Input: part model. Units: mm. Frame: model coordinates. Give positions to 0.01 mm unless a question says otherwise; leave off trailing zeros. Loops run counter-clockwise (first coordinate to the right, second up) from the corner with the lowest first, then second, coordinate; pieces in that order, holes last. Notation, with made-up numbers: (-18.5, 51.25) -> (16.5, 51.25) arc R28 cw to (16.5, 75.25) -> close; hole circle Ø3 at (13, -36). An arc over 180 degrees is marked (long way). Answer as a JSON object with one key per item and string values. Group by question number.
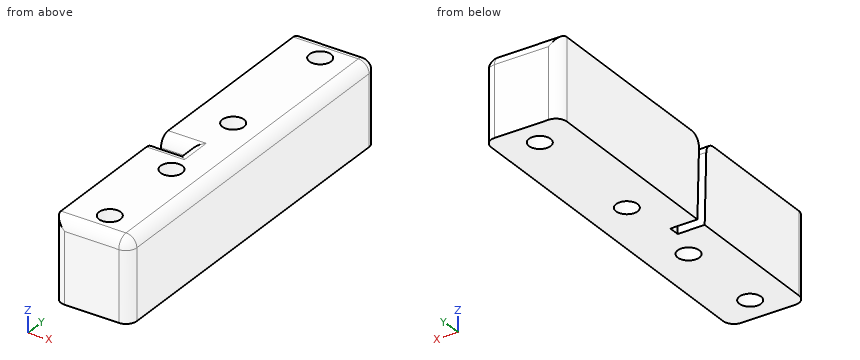
```python
from build123d import *

# Parameters (mm, degrees)
F0_W     = 14
F0_H     = 28
F0_R     = 2
F1_DEPTH = 15
F0_H_2   = 38
F2_W     = 2.6328479201
F2_H     = 15
F3_DEPTH = 9
F5_DEPTH = 5
F7_DEPTH = 5
F8_R     = 2


with BuildPart() as f1:
    # F0 (on Top) → F1 (new body)
    with BuildSketch(Plane.XY):
        with Locations((7, 14)):
            Rectangle(F0_W, F0_H)
        with Locations((7, 5)):
            Circle(F0_R, mode=Mode.SUBTRACT)
        with Locations((7, 22)):
            Circle(F0_R, mode=Mode.SUBTRACT)
    extrude(amount=F1_DEPTH)



with BuildPart() as f1b:
    # F0 (on Top) → F1, piece 2 (new body)
    with BuildSketch(Plane.XY):
        with Locations((7, 49)):
            Rectangle(F0_W, F0_H_2)
        with Locations((7, 39)):
            Circle(F0_R, mode=Mode.SUBTRACT)
        with Locations((7, 63)):
            Circle(F0_R, mode=Mode.SUBTRACT)
    extrude(amount=F1_DEPTH)


with BuildPart() as f1_1:
    add(f1.part)

    add(f1b.part)  # F3 merges F1b
    # F2 (on face) → F3 (join)
    with BuildSketch(Plane.YZ.offset(14)):
        with Locations((29.31642396, 7.5)):
            Rectangle(F2_W, F2_H)
    extrude(amount=-F3_DEPTH)

    # F4 (on face) → F5 (cut)
    with BuildSketch(Plane(origin=(0, 0, 0), x_dir=(0, -1, 0), z_dir=(-1, 0, 0))):
        Polygon((-28, 15), (-28, 0), (-27.5, 15), align=None)
    extrude(amount=-F5_DEPTH, mode=Mode.SUBTRACT)

    # F6 (on face) → F7 (join)
    with BuildSketch(Plane(origin=(0, 0, 0), x_dir=(0, -1, 0), z_dir=(-1, 0, 0))):
        Polygon((-29.5, 15), (-30, 15), (-30, 0), align=None)
    extrude(amount=-F7_DEPTH)

    # F8
    f8_edges = [f1_1.edges().sort_by_distance(p)[0] for p in [
        (2.5, 29.5, 15),
        (5, 28.5, 15),
        (2.5, 27.5, 15),
        (7, 0, 15),
        (14, 34, 15),
        (7, 68, 15),
        (14, 0, 7.5),
        (14, 68, 7.5),
        (0, 68, 7.5),
        (0, 0, 7.5),
    ]]
    fillet(f8_edges, radius=F8_R)


solid = f1_1.part
```
Q1. Ray query, probe 1 along Y at (x, z) = (7, 11.75); probe 2 along Y at (x, z) = (8.5, 3.5); probe 3 along Y at (x, z) = (4.75, 3.5). Return the intervals inside material, ascending.
Q2. Pin query (flat end, axial travel): pin 1 Ø1.2 at (y, z) = (29, 9.5) entering from -X. Return the tip coordinate at first contact, or that it passes through.
Q3. Section A-A on y = 63. Return the cut outline in (x, z), then the cut area to 3 significant figures.
Q4. Section C-C on x = 8. Return the cut outline in (y, z).
Q5. Section B-B on z = 4.75. Return the cut outline in (x, y).
Numbers:
{
 "1": {"probe 1": "y = 0 to 3, 7 to 20, 24 to 37, 41 to 61, 65 to 68", "probe 2": "y = 0 to 3.68, 6.32 to 20.68, 23.32 to 37.68, 40.32 to 61.68, 64.32 to 68", "probe 3": "y = 0 to 27.88, 29.88 to 68"},
 "2": {"pin 1": "stops at x = 5"},
 "3": {"outline": "(0, 0) -> (5, 0) -> (5, 15) -> (0, 15) -> close; (9, 0) -> (14, 0) -> (14, 13) arc R2 ccw to (12, 15) -> (9, 15) -> close", "area": "149 mm²"},
 "4": {"outline": "(0, 0) -> (3.27, 0) -> (3.27, 15) -> (2, 15) arc R2 ccw to (0, 13) -> close; (6.73, 0) -> (20.27, 0) -> (20.27, 15) -> (6.73, 15) -> close; (23.73, 0) -> (37.27, 0) -> (37.27, 15) -> (23.73, 15) -> close; (40.73, 0) -> (61.27, 0) -> (61.27, 15) -> (40.73, 15) -> close; (64.73, 0) -> (68, 0) -> (68, 13) arc R2 ccw to (66, 15) -> (64.73, 15) -> close"},
 "5": {"outline": "(0, 2) arc R2 ccw to (2, 0) -> (12, 0) arc R2 ccw to (14, 2) -> (14, 66) arc R2 ccw to (12, 68) -> (2, 68) arc R2 ccw to (0, 66) -> (0, 29.84) -> (5, 29.84) -> (5, 27.84) -> (0, 27.84) -> close; hole circle Ø4 at (7, 5); hole circle Ø4 at (7, 22); hole circle Ø4 at (7, 39); hole circle Ø4 at (7, 63)"}
}
